Verification items for the finished model (mm, model axes). Face numbers are marked on the shaded views. Coordinates: 2 decimals unless noted, no trailing zeros. Write each loop counter-clockwise with the first axis right and the second up, starting at its lowest first coordinate (ties: lowest second). Pieces come first, ordered by that corner, then holes. Notation, with made-up numbers: (13, 43.5) -> (60, 43.5) arc R27 cw to (60, 59.5) -> close; hole circle Ø4 at (-19, -10). An arc over 180 degrees is marked (long way). Use a Markdown table: item, result. Add a question column.
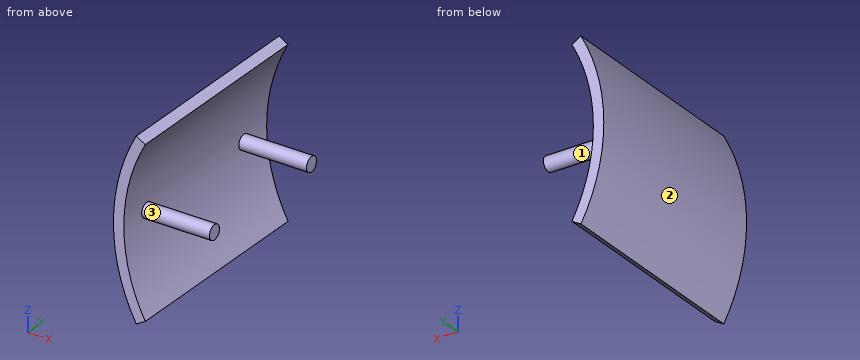
Autodesk Inventor part; units mm, degrees
ref_plane "YZ Plane" through (0, 0, 0) normal (1, 0, 0) x (0, 1, 0)
ref_plane "XZ Plane" through (0, 0, 0) normal (0, 1, 0) x (-1, 0, 0)
ref_plane "XY Plane" through (0, 0, 0) normal (0, 0, 1) x (1, 0, 0)
sketch "Sketch1" plane through (0, 0, 0) normal (0, 1, 0) x (-1, 0, 0)
  arc A0 (-87.5, 0) -> (0, 87.5) centre (0, 0) ccw
  arc A1 (-82.5, 0) -> (0, 82.5) centre (0, 0) ccw
  line L0 (0, 87.5) -> (0, 82.5)
  line L1 (-82.5, 0) -> (-87.5, 0)
  dimension "d0" = 165
  dimension "d1" = 175
  dimension "d7" = 0
  dimension "d8" = 0
extrude "Extrusion1" add sketch "Sketch1" along normal mid plane 100
sketch "Sketch5" plane through (0, 0, 0) normal (1, 0, 0) x (0, 1, 0)
  line L0 (-50, 0) -> (50, 0)
  circle A0 centre (34, 0) radius 3.5
  circle A1 centre (-34, 0) radius 3.5
  point P0 (0, 0)
  dimension "d22" = 7
  dimension "d23" = 7
  dimension "d24" = 68
  dimension "d25" = 34
extrude "Extrusion4" add sketch "Sketch5" against normal up to next
sketch "Sketch6" plane through (0, 34, 0) normal (1, 0, 0) x (0, 0, -1)
  circle A0 centre (0, 0) radius 3.5
  line L0 (0, -84) -> (0, 16)
  circle A1 centre (0, -68.0281) radius 3.5281
  point P0 (0, -34)
extrude "Extrusion5" cut sketch "Sketch6" against normal blind 50
sketch "Sketch7" plane through (0, 50, 0) normal (0, 1, 0) x (1, 0, 0)
  arc A0 (87.5, 0) -> (0, -87.5) centre (0, 0) ccw construction
  arc A1 (82.5, 0) -> (0, -82.5) centre (0, 0) ccw construction
  arc A2 (-87.5, 0) -> (-76.5573, -42.3702) centre (0, 0) ccw
  arc A3 (-82.5, 0) -> (-72.2264, -39.8698) centre (0, 0) ccw
  line L0 (-72.2264, -39.8698) -> (-76.5573, -42.3702)
  line L1 (0, 0) -> (-87.5, 0) construction
  arc A4 (0, 87.5) -> (87.5, 0) centre (0, 0) ccw construction
  arc A5 (0, 82.5) -> (82.5, 0) centre (0, 0) ccw construction
  arc A6 (-76.5573, 42.3702) -> (-87.5, 0) centre (0, 0) ccw
  arc A7 (-72.2264, 39.8698) -> (-82.5, 0) centre (0, 0) ccw
  line L2 (-72.2264, 39.8698) -> (-76.5573, 42.3702)
  arc A8 (82.5, 0) -> (-72.2264, 39.8698) centre (0, 0) ccw
  arc A9 (87.5, 0) -> (-76.5573, 42.3702) centre (0, 0) ccw
  arc A10 (-76.5573, -42.3702) -> (0, -87.5) centre (0, 0) ccw
  arc A11 (-72.2264, -39.8698) -> (0, -82.5) centre (0, 0) ccw
  line L3 (-156.1445, -133.794) -> (99.266, -133.794)
  line L4 (99.266, -133.794) -> (99.266, 159.7464)
  line L5 (99.266, 159.7464) -> (-156.1445, 159.7464)
  line L6 (-156.1445, 159.7464) -> (-156.1445, -133.794)
  circle A12 centre (0, 0) radius 82.5
  point P0 (0, -82.5)
  dimension "d30" = 30
  dimension "d31" = 45.3349
  dimension "d32" = 0
  dimension "d33" = 255.4104
  dimension "d34" = 293.5404
  dimension "d35" = 159.7464
  dimension "d36" = 11.766
extrude "Extrusion6" cut sketch "Sketch7" against normal up to next
sketch "Sketch3" plane through (0, 0, 0) normal (1, 0, 0) x (0, 1, 0)
  circle A0 centre (0, 34) radius 3.5
  circle A1 centre (0, -34) radius 3.5
  circle A2 centre (0, 34) radius 3.5
  circle A3 centre (0, -34) radius 3.5
  point P0 (0, 0)
  dimension "d9" = 7
  dimension "d10" = 7
  dimension "d11" = 68
  dimension "d12" = 34
  dimension "d13" = 34
sketch "Sketch4" plane through (0, 0, 34) normal (1, 0, 0) x (0, 0, -1)
  circle A0 centre (0, 0) radius 3.5
  circle A1 centre (68, 0) radius 3.5
  circle A2 centre (68, 0) radius 3.5
  point P0 (34, 0)
equation "\"d26\" = d23"
properties part number "airframe"
1) Thickness scan on L1, parallel to Z at x = -73, y = 34; L2, parallel to X at y = -41, z = 1.5; L3, parallel to X at y = -43, z = 24. Record the ranges inside material, lowest first.
2) Cross-section at C-C on x = -84. Record the boundary of the cut face in (y, z), then the cut area to 3 significant figures.
3) Cross-section at D-D on y = 34. Record the boundary of the cut face in (x, z).
4) Cross-section at A-A on x = -67. Record the boundary of the cut face in (y, z).
5) Gauge pin test, flat ends, axial feed: pin 1 (8 mm diameter, centred on y = -39, z = 19, fed in from +X); pin 2 (10 mm diameter, centred on y = -21, z = 3, fed in from +X); pin 3 (8 mm diameter, centred on y = -6.5, z = 13.5, fed in from -X); pin 4 (10 mm diameter, centred on x = -64, y = 21.5, fed in from +Z). Record the tip position at first contact, or that the pin passes through.
6) Cross-section at B-B on z = 0. Record the boundary of the cut face in (x, y).
7) Release check for a two-part mould opening along Y. For the marked faces 1, 2 and 3 record: released by +Y, released by -Y, zero draft, split by the parting line, or undercut.
Returned:
| question | item | result |
|---|---|---|
| 1 | L1 | z = -40.32 to -38.44, -3.5 to 3.5, 38.44 to 40.32 |
| 1 | L2 | x = -87.49 to -82.49 |
| 1 | L3 | x = -84.14 to -78.93 |
| 2 | outline | (-50, -24.5) -> (50, -24.5) -> (50, 24.5) -> (-50, 24.5) -> close |
| 2 | area | 4,900 mm² |
| 3 | outline | (-82.43, -3.5) -> (-50, -3.5) -> (-50, 3.5) -> (-82.43, 3.5) arc R82.5 cw to (-72.23, 39.87) -> (-76.56, 42.37) arc R87.5 ccw to (-76.56, -42.37) -> (-72.23, -39.87) arc R82.5 cw to start |
| 4 | outline | circle Ø7 at (-34, 0); circle Ø7 at (34, 0) |
| 5 | pin 1 | stops at x = -79.23 |
| 5 | pin 2 | stops at x = -82.11 |
| 5 | pin 3 | stops at x = -86.98 |
| 5 | pin 4 | passes through |
| 6 | outline | (-87.5, -50) -> (-82.5, -50) -> (-82.5, -37.5) -> (-50, -37.5) -> (-50, -30.5) -> (-82.5, -30.5) -> (-82.5, 30.5) -> (-50, 30.5) -> (-50, 37.5) -> (-82.5, 37.5) -> (-82.5, 50) -> (-87.5, 50) -> close |
| 7 | face 1 | undercut |
| 7 | face 2 | zero draft |
| 7 | face 3 | undercut |
